```python
from build123d import *

# Parameters (mm, degrees)
F0_R        = 3.175
F0_W        = 11.43
F0_H        = 35.56
F0_W_2      = 35.56
F0_H_2      = 10.9884785938
F1_DEPTH    = 3.81
F2_DEPTH    = 15.24
F3_T1_DEPTH = 35.56
F3_T3_DEPTH = 35.56


# Not quite as in the source:
# - a fillet or chamfer that OpenCascade refuses, or shapes differently, is made with other operations: its cross-section is extruded or revolved along the edge and cut away or added


with BuildPart() as f1:
    # F0 (on Front) → F1 (new body)
    with BuildSketch(Plane.XZ):
        with BuildLine():
            Line((246.8790987015, 3.8439502823), (5.5790987015, 3.8439502823))
            ThreePointArc((5.5790987015, 3.8439502823), (1.0889706409, 1.9840783429), (-0.7709012985, -2.5060497177))
            Line((-0.7709012985, -2.5060497177), (-0.7709012985, -196.0790987015))
            ThreePointArc((-0.7709012985, -196.0790987015), (0.1888954325, -198.3962529867), (2.5060497177, -199.3560497177))
            Line((2.5060497177, -199.3560497177), (246.8790987015, -199.3560497177))
            ThreePointArc((246.8790987015, -199.3560497177), (251.369226762, -197.4961777782), (253.2290987015, -193.0060497177))
            Line((253.2290987015, -193.0060497177), (253.2290987015, -2.5060497177))
            ThreePointArc((253.2290987015, -2.5060497177), (251.369226762, 1.9840783429), (246.8790987015, 3.8439502823))
        make_face()
        with Locations((18.2790987015, -139.0930234075)):
            Circle(F0_R, mode=Mode.SUBTRACT)
        with Locations((234.1790987015, -189.8930234075)):
            Circle(F0_R, mode=Mode.SUBTRACT)
        with Locations((227.8290987015, -184.0757250905)):
            Circle(F0_R, mode=Mode.SUBTRACT)
        with BuildLine():
            ThreePointArc((232.1718121719, -113.6930234075), (237.2518121719, -108.6130234075), (242.3318121719, -113.6930234075))
            ThreePointArc((242.3318121719, -113.6930234075), (237.2518121719, -118.7730234075), (232.1718121719, -113.6930234075))
        make_face(mode=Mode.SUBTRACT)
        with Locations((18.2790987015, -88.2930234075)):
            Circle(F0_R, mode=Mode.SUBTRACT)
        with Locations((164.6692329311, -23.1037478608)):
            Rectangle(F0_W, F0_H, mode=Mode.SUBTRACT)
        with Locations((227.8290987015, -44.3757250905)):
            Circle(F0_R, mode=Mode.SUBTRACT)
        with Locations((234.1790987015, -37.4930234075)):
            Circle(F0_R, mode=Mode.SUBTRACT)
        with Locations((202.1326256323, -10.8179871577)):
            Rectangle(F0_W_2, F0_H_2, mode=Mode.SUBTRACT)
        with Locations((164.6692329311, -23.1037478608)):
            Rectangle(F0_W, F0_H)
        with Locations((202.1326256323, -10.8179871577)):
            Rectangle(F0_W_2, F0_H_2)
    extrude(amount=F1_DEPTH)

    # F0 (on Front) → F2 (join)
    with BuildSketch(Plane.XZ):
        with Locations((164.6692329311, -23.1037478608)):
            Rectangle(F0_W, F0_H)
        with Locations((202.1326256323, -10.8179871577)):
            Rectangle(F0_W_2, F0_H_2)
    extrude(amount=F2_DEPTH)

    # F3: fillet of radius 5.588 on 4 edges, made by hand

    # F3_s2 → F3_t1 (cut)
    with BuildSketch(Plane.XY.offset(-40.8837478608)):
        with BuildLine():
            ThreePointArc((158.9542329311, -9.652), (160.5909202379, -13.6033126933), (164.5422329311, -15.24))
            Line((164.5422329311, -15.24), (164.5422329311, -15.35176))
            Line((164.5422329311, -15.35176), (158.8424729311, -15.35176))
            Line((158.8424729311, -15.35176), (158.8424729311, -9.652))
            Line((158.8424729311, -9.652), (158.9542329311, -9.652))
        make_face()
        with BuildLine():
            ThreePointArc((170.3842329311, -9.652), (168.7475456244, -13.6033126933), (164.7962329311, -15.24))
            Line((164.7962329311, -15.24), (164.7962329311, -15.35176))
            Line((164.7962329311, -15.35176), (170.4959929311, -15.35176))
            Line((170.4959929311, -15.35176), (170.4959929311, -9.652))
            Line((170.4959929311, -9.652), (170.3842329311, -9.652))
        make_face()
    extrude(amount=F3_T1_DEPTH, mode=Mode.SUBTRACT)

    # F3_s4 → F3_t3 (cut)
    with BuildSketch(Plane.YZ.offset(184.3526256323)):
        with BuildLine():
            ThreePointArc((-9.652, -5.3237478608), (-13.6033126933, -6.9604351675), (-15.24, -10.9117478608))
            Line((-15.24, -10.9117478608), (-15.35176, -10.9117478608))
            Line((-15.35176, -10.9117478608), (-15.35176, -5.2119878608))
            Line((-15.35176, -5.2119878608), (-9.652, -5.2119878608))
            Line((-9.652, -5.2119878608), (-9.652, -5.3237478608))
        make_face()
        with BuildLine():
            ThreePointArc((-9.652, -16.3122264546), (-13.6033126933, -14.6755391479), (-15.24, -10.7242264546))
            Line((-15.24, -10.7242264546), (-15.35176, -10.7242264546))
            Line((-15.35176, -10.7242264546), (-15.35176, -16.4239864546))
            Line((-15.35176, -16.4239864546), (-9.652, -16.4239864546))
            Line((-9.652, -16.4239864546), (-9.652, -16.3122264546))
        make_face()
    extrude(amount=F3_T3_DEPTH, mode=Mode.SUBTRACT)


solid = f1.part
```
Geometry: final body of the model. Coordinates: model frame, mm. A direction names the side the tool comes from. Round coordinates to 2 decimals unless told otherwise and drop trailing zeros. Order: outer loops, then holes, each group sorted by start corner. A loop starts at its lowest first (then second) coordinate and runs counter-clockwise, first axis right, second up. Notation, with made-up numbers: (24, 14) - (69, 14) arc R24 ccw to (69, 30) - close; hole circle Ø8 at (13, 87). An arc over 180 degrees is marked (long way). Write item = value, one per line. Start each with the question number.
Q1. Cut plane A-A on x = 196. Return the cut outline in (y, z), and give its area (3 significant figures).
Q2. Pin query (flat end, axial travel): pin 1 (11.5 mm diameter, centred on x = 237.25, z = -113.69, fed in from -Y); pin 2 (4 mm diameter, centred on x = 227.83, z = -184.08, fed in from -Y); pin 3 (3.5 mm diameter, centred on x = 163, y = -8, fed in from +Z); pin 4 (3.5 mm diameter, centred on x = 164, y = -8, fed in from -Z). Return the tip coordinate at first contact, or that it passes through.
Q3. Cut plane B-B on z = -82. Return the cut outline in (x, y).
Q4. Access query for faces 1 (the cylindrical face through (201.88, -13.53, -6.89)), 2 (the flat face through (219.913, -9, -11)), 3 (the flat face through (202, -7, -16.312)), 4 (the flat face through (184.353, -9, -11)). Directions: +Z, -Z, +X, -X, +Y, -Y. A direction counts if a zero-diameter tool reaches every point of the face in a straight line with its end or side. Return the directions, or none.
Q5. Cut plane C-C on x = 65.5. Return the cut outline in (y, z).
Q6. Pull-direction query (X, two-part tool) for faces 5 (the cylindrical face through (251.32, -1.878, -197.545)), 6 (the flat face through (165, -9, -5.324)), 7 (the cylindrical face through (233.51, -1.88, -117.13)); classes: +X half, -X half, draft (parallel to the pull), parting line (faces both ways), or undercut.
Q7. Ray query, line 1 (Y direction, x = 143, z = -113); line 2 (Z direction, x = 165, y = -5); line 3 (Z direction, x = 188.5, y = -11.5). Return the intervals inside material, ascending. Write a range as from..to.
Outcome:
q1.outline = (-15.24, -10.82) arc R5.59 ccw to (-9.65, -16.31) - (-3.81, -16.31) - (-3.81, -199.36) - (0, -199.36) - (0, 3.84) - (-3.81, 3.84) - (-3.81, -5.32) - (-9.65, -5.32) arc R5.59 ccw to start
q1.area = 886 mm^2
q2.pin_1 = -3.81
q2.pin_2 = through
q2.pin_3 = -5.32
q2.pin_4 = -40.88
q3.outline = (-0.77, -3.81) - (253.23, -3.81) - (253.23, 0) - (-0.77, 0) - close
q4.face_1 = +Z, +X, -Y
q4.face_2 = +Z, -Z, +X, -Y
q4.face_3 = -Z, +X, -Y
q4.face_4 = +Z, -Z, -Y
q5.outline = (-3.81, -199.36) - (0, -199.36) - (0, 3.84) - (-3.81, 3.84) - close
q6.face_5 = +X half
q6.face_6 = draft
q6.face_7 = undercut
q7.line_1 = -3.81..0
q7.line_2 = -40.88..-5.32
q7.line_3 = -16..-5.64
